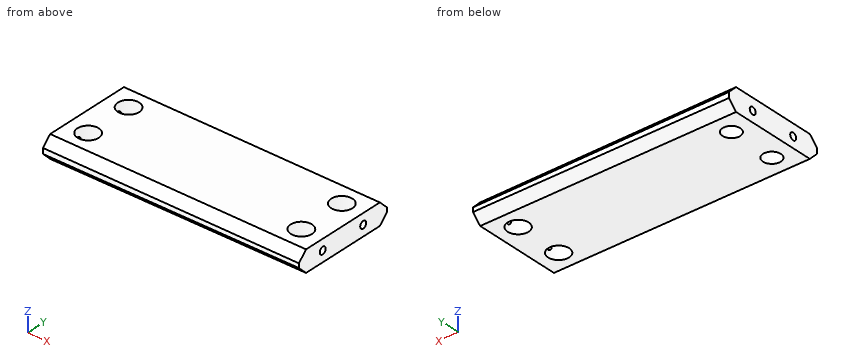
```python
from build123d import *

# Parameters (mm, degrees)
BOSS_EXTRUDE3_DEPTH                  = 46.99
CHAMFER1_SIZE                        = 7.62
F_3_4_0_75_DIAMETER_HOLE1_AT_2_COUNT = 2
F_3_4_0_75_DIAMETER_HOLE1_AT_2_PITCH = 190.5


with BuildPart() as part:
    # 3DSketch2 → Boss-Extrude3 (new, symmetric)
    with BuildSketch(Plane(origin=(-117.411769765, 0, -9.784420547), x_dir=(0.9965456835069088, 0, 0.08304637670451492), z_dir=(0, -1, 0))):
        Polygon((0, 0), (227.81034325, -18.984401715), (229.389897471, 0), (1.670602813, 20.047015755), align=None)
    extrude(amount=BOSS_EXTRUDE3_DEPTH, both=True)

    # Chamfer1
    chamfer1_edges = [part.edges().sort_by_distance(p)[0] for p in [
        (-3.111769765, 46.99, -9.784420547),
        (-3.113013683, -46.99, 9.798831636),
        (-3.111769765, -46.99, -9.784420547),
        (-3.113013683, 46.99, 9.798831636),
    ]]
    chamfer(chamfer1_edges, length=CHAMFER1_SIZE)

    # Sketch3 → 3/4 (0.75) Diameter Hole1 (revolve, cut)
    with BuildSketch(Plane(origin=(92.135949719, -21.59, 9.354454682), x_dir=(0.9999891170795402, 0, -0.0046653748490357765), z_dir=(0, 1, 0))):
        Polygon((0, 0), (0, 24.773197396), (9.525, 19.05), (9.525, 0), align=None)
    f_3_4_0_75_diameter_hole1 = revolve(axis=Axis((92.165574849, -21.59, 15.704385575), (-0.004665374849035791, 0, -0.9999891170795401)), mode=Mode.SUBTRACT)

    # 3/4 (0.75) Diameter Hole1 at 2: 3/4 (0.75) Diameter Hole1 ×2
    with Locations(*[Vector(-0.9999891170795401, 0, 0.004665374849035796) * (i * F_3_4_0_75_DIAMETER_HOLE1_AT_2_PITCH) for i in range(1, F_3_4_0_75_DIAMETER_HOLE1_AT_2_COUNT)]):
        add(f_3_4_0_75_diameter_hole1, mode=Mode.SUBTRACT)

    # Sketch5 → 1/4 (0.25) Diameter Hole1 (revolve, cut)
    with BuildSketch(Plane(origin=(111.186986317, -21.59, -0.259420628), x_dir=(0.00013059504552427994, 0, -0.9999999914724671), z_dir=(0, 1, 0))):
        Polygon((0, 0), (0, 20.957732465), (3.175, 19.05), (3.175, 0), align=None)
    f_1_4_0_25_diameter_hole1 = revolve(axis=Axis((117.536986263, -21.59, -0.258591349), (-0.9999999914724671, 0, -0.00013059504552427964)), mode=Mode.SUBTRACT)

    # Sketch7 → 1/4 (0.25) Diameter Hole2 (revolve, cut)
    with BuildSketch(Plane(origin=(-117.411769765, -21.59, -0.259420547), x_dir=(0, 0, 1), z_dir=(0, 1, 0))):
        Polygon((0, 0), (0, 20.957732465), (3.175, 19.05), (3.175, 0), align=None)
    f_1_4_0_25_diameter_hole2 = revolve(axis=Axis((-123.761769765, -21.59, -0.259420547), (1, 0, 0)), mode=Mode.SUBTRACT)

    # Mirror9: 3/4 (0.75) Diameter Hole1, 1/4 (0.25) Diameter Hole1, 1/4 (0.25) Diameter Hole2 across plane
    add(f_3_4_0_75_diameter_hole1.mirror(Plane.ZX), mode=Mode.SUBTRACT)
    add(f_1_4_0_25_diameter_hole1.mirror(Plane.ZX), mode=Mode.SUBTRACT)
    add(f_1_4_0_25_diameter_hole2.mirror(Plane.ZX), mode=Mode.SUBTRACT)

    # Mirror9 copy 1 sketch → Mirror9 copy 1 (revolve, cut)
    with BuildSketch(Plane(origin=(-98.361977085, 21.59, 10.24320859), x_dir=(0.9999891170795402, 0, -0.0046653748490357765), z_dir=(0, -1, 0))):
        Polygon((0, 0), (0, -24.773197396), (9.525, -19.05), (9.525, 0), align=None)
    revolve(axis=Axis((-98.332351955, 21.59, 16.593139484), (0.004665374849035791, 0, 0.9999891170795401)), mode=Mode.SUBTRACT)


solid = part.part
```
Here's how the part is built. I have some questions about the finished solid (model axes, mm). Coordinates: 2 decimals unless noted, no trailing zeros. Loops run counter-clockwise (first coordinate to the right, second up) from the corner with the lowest first, then second, coordinate; pieces in that order, holes last. Notation, with made-up numbers: (43.25, 36.5) - (79.25, 36.5) arc R14 ccw to (79.25, 53.5) - close; hole circle Ø2 at (6.25, 76). An arc over 180 degrees is marked (long way). Return JSON: item names as keys, results as strings. Group by question number.
Item 1: If we section it at B-B on x = -80: Write out the boundary of the cut face in (y, z).
Item 2: If we section it at C-C on z = 5.25: State how many separate pieces and enclosed holes the cut face has, and give its area (3 significant figures).
Item 3: If we section it at A-A on y = 21.59: Write out the boundary of the cut face in (x, z), and give its area (3 significant figures).
Item 4: Will these pins go through, and if not, where does the flat tip stop? P1, Ø10, axis at x = 56.5, z = 5, coming from the +Y side; P2, Ø5, axis at y = 21.59, z = -0.26, coming from the -X side; P3, Ø10, axis at x = 12.5, y = 29, coming from the +Z side; P4, Ø4, axis at y = -21.59, z = -0.26, coming from the -X side.
Item 5: I need wall thicknesses on line 1 (Z direction, x = 105.5, y = -21.59); line 2 (X direction, y = 16, z = 5.75); line 3 (Y direction, x = -106.5, z = 5). Which ranges of each line are inside material? Lowest first, please. Write a range as from..to.
Item 6: If we section it at D-D on x = 35: Write out the boundary of the cut face in (y, z), and give its area (3 significant figures).
Calculated:
{
 "1": {"outline": "(-46.99, -2.16) - (-39.37, -9.78) - (39.37, -9.78) - (46.99, -2.16) - (46.99, 2.54) - (39.37, 10.16) - (-39.37, 10.16) - (-46.99, 2.54) - close"},
 "2": {"separate pieces": "1", "enclosed holes": "4", "area": "18,900 mm^2"},
 "3": {"outline": "(-117.41, -9.78) - (-106.29, -9.78) - (-107.98, -8.76) - (-107.95, -3.43) - (-117.41, -3.43) - close; (-117.41, 2.92) - (-107.92, 2.92) - (-107.89, 10.29) - (-117.41, 10.33) - close; (-90.5, -9.78) - (82.74, -9.78) - (82.52, -9.65) - (82.61, 9.4) - (-88.84, 10.2) - (-88.93, -8.85) - close; (101.5, -9.78) - (111.19, -9.78) - (111.19, -3.43) - (101.6, -3.44) - (101.57, -9.74) - close; (101.63, 2.91) - (111.19, 2.92) - (111.19, 9.27) - (101.66, 9.31) - close", "area": "3,610 mm^2"},
 "4": {"P1": "stops at y = 46.99", "P2": "stops at x = -89.22", "P3": "stops at z = 9.75", "P4": "stops at x = -89.1"},
 "5": {"line 1": "z = -9.78..-3.44, 2.91..9.29", "line 2": "x = -117.41..-106.1, -90.67..84.41, 99.83..111.19", "line 3": "y = -44.65..-26.58, -16.6..16.6, 26.58..44.65"},
 "6": {"outline": "(-46.99, -2.16) - (-39.37, -9.78) - (39.37, -9.78) - (46.99, -2.16) - (46.99, 2) - (39.37, 9.62) - (-39.37, 9.62) - (-46.99, 2) - close", "area": "1,710 mm^2"}
}
